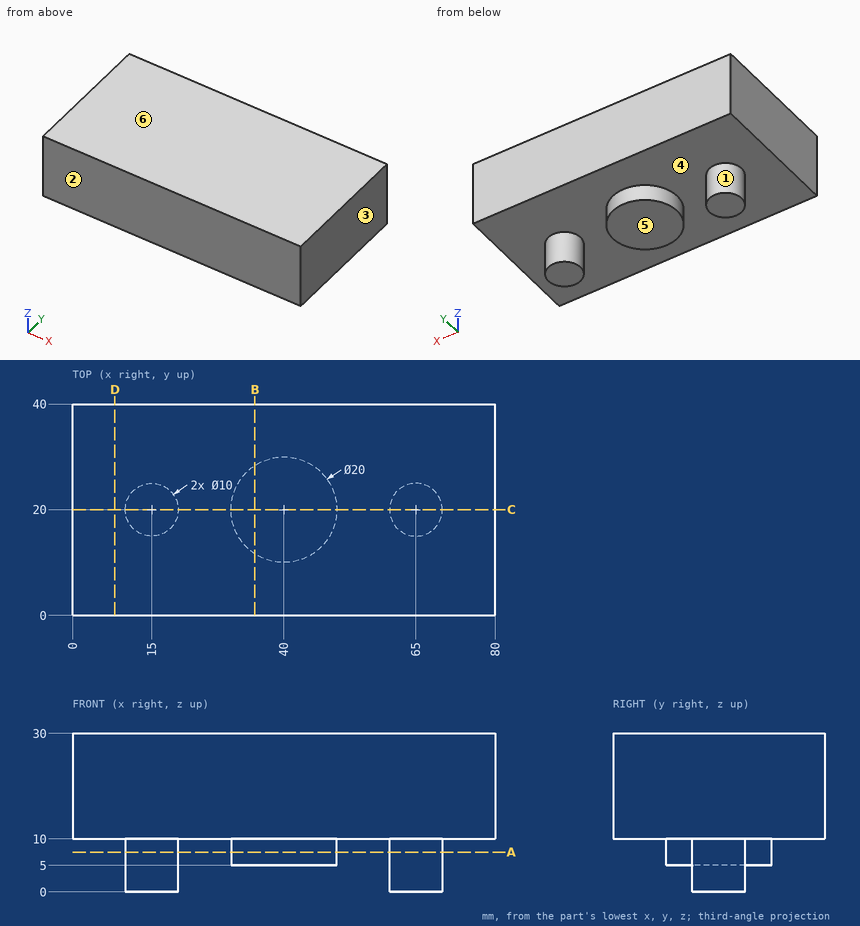
Study the drawing (mm; zero at the part's minimum x, y, z) and answer. A direction names the side the tool comes from. Give positions to 0.01 mm unless a question says otherwise; leave off trailing zeros. Write each loop counter-clockwise with the first axis right and the second up, starting at its lowest first coordinate (ties: lowest second). Pieces come first, ordered by that corner, then holes. Notation, with made-up numbers: (-21.5, 24) -> (-10.5, 24) arc R32 ccw to (-10.5, 56) -> close; hole circle Ø5 at (60.5, 68). An arc over 180 degrees is marked (long way). Write item = value, one per line. Start each with the question number.
1) Determine the mould class of the marked faces 1, 2 and 3 for opening direction X: +X half, -X half, draft (parallel to the pull), parting line (faces both ways), or undercut.
2) The part is cut by section C-C, the plane y = 20. Determine the outline of the cut face in (x, z).
3) Straight lines are drawn through the part: line 1 along Z through (x, y) = (47, 22); line 2 along Z through (x, y) = (58, 31); line 3 along Y through (x, z) = (31.5, 8.5). For each, find the intervals that lie inside material, in ascending order.
4) Which of the six approach directions +Z, -Z, +X, -X, +Y, -Y give full straight-line access (tool end or side, diameter ignored) to the marked faces 4, 5 and 6?
5) The part is cut by section D-D, the plane x = 8. Determine the outline of the cut face in (y, z), and give its area (3 significant figures).
6) The part is cut by section A-A, the plane z = 7.5. Determine the outline of the cut face in (x, y).
7) The part is cut by section B-B, the plane x = 34.5. Determine the outline of the cut face in (y, z).
8) Each of these flat-tipped pins is pushed along its axis until it touches: pin 1 (2 mm diameter, centred on x = 16.5, z = 6, fed in from +Y); pin 2 (16 mm diameter, centred on x = 38, y = 20, fed in from -Z); pin 3 (1 mm diameter, centred on y = 17, z = 9, fed in from +X). Where does it stop, or does it pass through?
Solutions:
q1.face_1 = undercut
q1.face_2 = draft
q1.face_3 = +X half
q2.outline = (0, 10) -> (10, 10) -> (10, 0) -> (20, 0) -> (20, 10) -> (30, 10) -> (30, 5) -> (50, 5) -> (50, 10) -> (60, 10) -> (60, 0) -> (70, 0) -> (70, 10) -> (80, 10) -> (80, 30) -> (0, 30) -> close
q3.line_1 = 5 to 30
q3.line_2 = 10 to 30
q3.line_3 = 14.73 to 25.27
q4.face_4 = -Z
q4.face_5 = -Z, +Y, -Y
q4.face_6 = +Z, +X, -X, +Y, -Y
q5.outline = (0, 10) -> (40, 10) -> (40, 30) -> (0, 30) -> close
q5.area = 800 mm²
q6.outline = circle Ø10 at (15, 20); circle Ø20 at (40, 20); circle Ø10 at (65, 20)
q7.outline = (0, 10) -> (11.65, 10) -> (11.65, 5) -> (28.35, 5) -> (28.35, 10) -> (40, 10) -> (40, 30) -> (0, 30) -> close
q8.pin_1 = 24.97
q8.pin_2 = 5
q8.pin_3 = 69.33
